Verification items for the finished model (mm, model axes). A direction names the side the tool comes from. Coordinates: 2 decimals unless noted, no trailing zeros. Loops run counter-clockwise (first coordinate to the right, second up) from the corner with the lowest first, then second, coordinate; pieces in that order, holes last. Notation, with made-up numbers: (25, 1) - (39, 1) arc R19 ccw to (39, 7) - close; hole circle Ø7 at (2, -37.75). An arc over 180 degrees is marked (long way). Answer as CSV lines item,"result". Start each with the question number.
1. Material ranges on line 1 (X direction, y = 26.25, z = 0); line 2 (X direction, y = 7, z = -19.5) (3 decimals); line 3 (X direction, y = 12, z = -19), recorded low to high. Write a range as [from, to].
2. Cross-section at A-A (x = 0). State how many separate pieces and enclosed holes the cut face has, plus the area to 3 significant figures.
3. Cross-section at D-D (y = 22.5). Enter the section's corners in (x, z).
4. Gauge pin test, flat ends, axial feed: P1, Ø6, axis at y = 21, z = 1.5, coming from the +X side; P2, Ø5, axis at x = 27.5, y = 6.5, coming from the +Z side; P3, Ø2, axis at x = 35, y = 15, coming from the -Z side. Record the tip position at first contact, or that the pin passes through.
5. Release check for a two-part mould opening along X. For faces 1 (the cylindrical face through (0.154, 9.86, 35.503)), 2 (the flat face through (-30.5, 0, -13.8)), 3 (the cylindrical face through (38.787, 9.86, 24.729)) record: pulls with the +X half, pulls with the -X half, needs draft (parallel to the pull), parting line crosses it, or undercut.
6. Cross-section at B-B (z = 0). Enter the section's corners in (x, y), plus the area to 3 significant figures.
7. Set-up check for faces 4 (the cylindrical face through (-6.834, 24.563, -1.517)), 5 (the cylindrical face through (39.284, 11.905, -0.867)), 6 (the cylindrical face through (-30.824, 9.86, 21.382)), 7 (the cylindrical face through (-32.215, 6.902, 7.154)): record each of +Z, -Z, +X, -X, +Y, -Y from which the full face is reachable in a straight line by a thin tool's end or side.
8. Cross-section at C-C (z = -39). Enter the section's corners in (x, y).
```python
from build123d import *

# Parameters (mm, degrees)
SKETCH1_R           = 46
SKETCH1_R_2         = 3.5
BOSS_EXTRUDE1_DEPTH = 20
SKETCH2_R           = 12
BOSS_EXTRUDE2_DEPTH = 10
SKETCH3_R           = 33
CUT_EXTRUDE1_DEPTH  = 14
SKETCH4_R           = 2.5
CUT_EXTRUDE2_DEPTH  = 6
SKETCH5_R           = 7
CUT_EXTRUDE3_DEPTH  = 10
CHAMFER2_SIZE       = 1
SKETCH6_R           = 4
CUT_EXTRUDE4_DEPTH  = 72.637978754


with BuildPart() as part:
    # Sketch1 → Boss-Extrude1 (new body)
    with BuildSketch(Plane(origin=(0, 0, 0), x_dir=(1, 0, 0), z_dir=(0, 1, 0))):
        with Locations(Location((0, 0, 0), (0, 0, 270))):
            Circle(SKETCH1_R)
        with Locations(Location((0, 39, 0), (0, 0, 270))):
            Circle(SKETCH1_R_2, mode=Mode.SUBTRACT)
        with Locations(Location((33.774990748, 19.5, 0), (0, 0, 270))):
            Circle(SKETCH1_R_2, mode=Mode.SUBTRACT)
        with Locations(Location((33.774990748, -19.5, 0), (0, 0, 270))):
            Circle(SKETCH1_R_2, mode=Mode.SUBTRACT)
        with Locations(Location((0, -39, 0), (0, 0, 270))):
            Circle(SKETCH1_R_2, mode=Mode.SUBTRACT)
        with Locations(Location((-33.774990748, -19.5, 0), (0, 0, 270))):
            Circle(SKETCH1_R_2, mode=Mode.SUBTRACT)
        with Locations(Location((-33.774990748, 19.5, 0), (0, 0, 270))):
            Circle(SKETCH1_R_2, mode=Mode.SUBTRACT)
    extrude(amount=BOSS_EXTRUDE1_DEPTH)

    # Sketch2 → Boss-Extrude2 (add)
    with BuildSketch(Plane(origin=(0, 20, 0), x_dir=(1, 0, 0), z_dir=(0, 1, 0))):
        with Locations(Location((0, 0, 0), (0, 0, 270))):
            Circle(SKETCH2_R)
    extrude(amount=BOSS_EXTRUDE2_DEPTH)

    # Sketch3 → Cut-Extrude1 (cut)
    with BuildSketch(Plane.XZ):
        with Locations(Location((0, 0, 0), (0, 0, 270))):
            Circle(SKETCH3_R)
    extrude(amount=-CUT_EXTRUDE1_DEPTH, mode=Mode.SUBTRACT)

    # Sketch4 → Cut-Extrude2 (cut)
    with BuildSketch(Plane.XZ.offset(-14)):
        with Locations(Location((0, 0, 0), (0, 0, 270))):
            Circle(SKETCH4_R)
    extrude(amount=-CUT_EXTRUDE2_DEPTH, mode=Mode.SUBTRACT)

    # Sketch5 → Cut-Extrude3 (cut)
    with BuildSketch(Plane(origin=(0, 30, 0), x_dir=(1, 0, 0), z_dir=(0, 1, 0))):
        with Locations(Location((0, 0, 0), (0, 0, 270))):
            Circle(SKETCH5_R)
    extrude(amount=-CUT_EXTRUDE3_DEPTH, mode=Mode.SUBTRACT)

    # Chamfer2
    chamfer2_edges = [part.edges().sort_by_distance(p)[0] for p in [
        (0, 30, -7),
    ]]
    chamfer(chamfer2_edges, length=CHAMFER2_SIZE)

    # Sketch6 → Cut-Extrude4 (cut, through all)
    with BuildSketch(Plane(origin=(0, 0, 0), x_dir=(0, 0, -1), z_dir=(1, 0, 0))):
        with Locations(Location((0, 8, 0), (0, 0, 180))):
            Circle(SKETCH6_R)
    extrude(amount=CUT_EXTRUDE4_DEPTH, mode=Mode.SUBTRACT)


solid = part.part
```
Values follow:
1,line 1,"x = [-12, -7], [7, 12]"
1,line 2,"x = [-41.662, -37.275], [-30.275, -26.622], [26.622, 30.275], [37.275, 41.662]"
1,line 3,"x = [-41.89, -37.24], [-30.31, -26.98], [26.98, 30.31], [37.24, 41.89]"
2,separate pieces,"4"
2,enclosed holes,"0"
2,area,"705 mm²"
3,outline,"circle Ø24 at (0, 0); hole circle Ø14 at (0, 0)"
4,P1,"stops at x = 46"
4,P2,"stops at z = 38.61"
4,P3,"stops at z = -30.98"
5,face 1,"undercut"
5,face 2,"needs draft"
5,face 3,"parting line crosses it"
6,outline,"(-46, 0) - (-33, 0) - (-33, 14) - (-2.5, 14) - (-2.5, 20) - (-7, 20) - (-7, 29) - (-8, 30) - (-12, 30) - (-12, 20) - (-46, 20) - close; (2.5, 14) - (33, 14) - (33, 12) - (46, 12) - (46, 20) - (12, 20) - (12, 30) - (8, 30) - (7, 29) - (7, 20) - (2.5, 20) - close; (33, 0) - (46, 0) - (46, 4) - (33, 4) - close"
6,area,"881 mm²"
7,face 4,"+Y"
7,face 5,"+X"
7,face 6,"+Y, -Y"
7,face 7,"-Y"
8,outline,"(-24.39, 0) - (-3.5, 0) - (-3.5, 20) - (-24.39, 20) - close; (3.5, 0) - (24.39, 0) - (24.39, 20) - (3.5, 20) - close"
